from build123d import *

# Parameters (mm, degrees)
SKETCH_1_R          = 11.2
EXTRUDE_1_DEPTH     = 2
SKETCH_2_OUTSIDE_W  = 30.748
SKETCH_2_OUTSIDE_H  = 30.748
CUT_EXTRUDE_1_DEPTH = 2
SKETCH_3_R          = 6.9
EXTRUDE_2_DEPTH     = 13.5
SKETCH_4_R          = 1.2
CUT_EXTRUDE_2_DEPTH = 13.5
FILLET_1_R          = 0.3


with BuildPart() as part:
    # 草图1 → 凸台-拉伸1 (new body)
    with BuildSketch(Plane(origin=(0, 0, 0), x_dir=(1, 0, 0), z_dir=(0, 1, 0))):
        with Locations(Location((0, 0, 0), (0, 0, 270))):
            Circle(SKETCH_1_R)
    extrude(amount=EXTRUDE_1_DEPTH)

    # 草图2 outside → 切除-拉伸1 (cut)
    with BuildSketch(Plane(origin=(0, 2, 0), x_dir=(1, 0, 0), z_dir=(0, 1, 0))):
        Rectangle(SKETCH_2_OUTSIDE_W, SKETCH_2_OUTSIDE_H)
        with BuildLine():
            Line((-8, -7.838367177), (8, -7.838367177))
            ThreePointArc((8, -7.838367177), (11.2, 0), (8, 7.838367177))
            Line((8, 7.838367177), (-8, 7.838367177))
            ThreePointArc((-8, 7.838367177), (-11.2, 0), (-8, -7.838367177))
        make_face(mode=Mode.SUBTRACT)
    extrude(amount=-CUT_EXTRUDE_1_DEPTH, mode=Mode.SUBTRACT)

    # 草图3 → 凸台-拉伸2 (add)
    with BuildSketch(Plane(origin=(0, 2, 0), x_dir=(1, 0, 0), z_dir=(0, 1, 0))):
        with Locations(Location((0, 0, 0), (0, 0, 270))):
            Circle(SKETCH_3_R)
    extrude(amount=EXTRUDE_2_DEPTH)

    # 草图4 → 切除-拉伸2 (cut)
    with BuildSketch(Plane(origin=(0, 2, 0), x_dir=(1, 0, 0), z_dir=(0, 1, 0))):
        with Locations(Location((-8, 5, 0), (0, 0, 270))):
            Circle(SKETCH_4_R)
        with Locations(Location((-8, -5, 0), (0, 0, 270))):
            Circle(SKETCH_4_R)
        with Locations(Location((8, -5, 0), (0, 0, 270))):
            Circle(SKETCH_4_R)
        with Locations(Location((8, 5, 0), (0, 0, 270))):
            Circle(SKETCH_4_R)
    extrude(amount=-CUT_EXTRUDE_2_DEPTH, mode=Mode.SUBTRACT)

    # 圆角1
    fillet_1_edges = [part.edges().sort_by_distance(p)[0] for p in [
        (0, 15.5, -6.9),
    ]]
    fillet(fillet_1_edges, radius=FILLET_1_R)

    # 草图5 → 切除-旋转1 (revolve, cut)
    with BuildSketch(Plane(origin=(0, 15.5, 0), x_dir=(1, 0, 0), z_dir=(0, 1, 0))):
        with BuildLine():
            Line((0, 4.5), (0, -4.5))
            ThreePointArc((0, -4.5), (4.5, 0), (0, 4.5))
        make_face()
    revolve(axis=Axis((0, 15.5, 4.5), (0, 0, -1)), mode=Mode.SUBTRACT)


solid = part.part
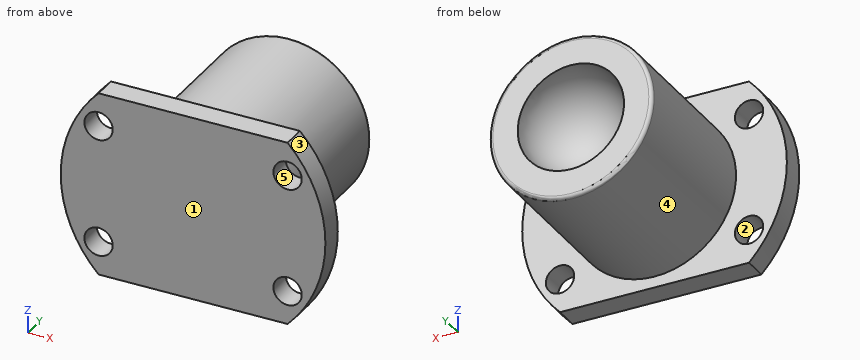
Here's how the part is built. I have some questions about the finished solid (model axes, mm). Face numbers are marked on the shaded views. A direction names the side the tool comes from. Coordinates: 2 decimals unless noted, no trailing zeros. Loops run counter-clockwise (first coordinate to the right, second up) from the corner with the lowest first, then second, coordinate; pieces in that order, holes last.
1. Imagine slicing it at A-A, the plane x = -8.5. Please give me the cut outline in (y, z).
2. Imagine slicing it at B-B, the plane z = 0. Please give me the cut outline in (x, y), and give its area (3 significant figures).
3. If we mould it in two halves opening along X, with no side actions, what happens to the marked faces 1, 2 and 3? For each: pulls with the +X half, pulls with the -X half, needs draft (parallel to the pull), parting line crosses it, or undercut.
4. For the marked faces 4 and 5, which set-ups out of +Z, -Z, +X, -X, +Y, -Y let a thin tool reach every point of the face, with its end or its side?
5. Imagine slicing it at D-D, the plane y = 14. Please give me the cut outline in (x, z).
6. I need wall thicknesses on L1, parallel to X at y = 1.35, z = -5; L2, parallel to Y at x = -1.75, z = 6.75; L3, parallel to X at y = 6.25, z = 0.25. Which ranges of each line are inside material? Lowest first, please.
7. Imagine slicing it at C-C, the plane y = 3. Please give me the cut outline in (x, z).
8. For P1, Ø4, axis at x = 8, z = 5, coming from the +Y side; P2, Ø1.5, axis at x = -2.5, y = 11.5, coming from the +Z side; P3, Ø5, axis at y = 10.5, z = -2.5, coming from the +X side; P4, Ø1.9, axis at x = 8, z = -5, coming from the -Y side, each with a flat end and sliding along its axis, tell me the tip position at first contact or that it passes through.
Taken from the geometry:
1. outline: (0, -7.29) - (2, -7.29) - (2, -6.09) - (0, -6.09) - close; (0, -3.91) - (2, -3.91) - (2, 3.91) - (0, 3.91) - close; (0, 6.09) - (2, 6.09) - (2, 7.29) - (0, 7.29) - close
2. outline: (-11.2, 0) - (11.2, 0) - (11.2, 2) - (6.9, 2) - (6.9, 15.2) arc R0.3 ccw to (6.6, 15.5) - (4.5, 15.5) arc R4.5 cw to (-4.5, 15.5) - (-6.6, 15.5) arc R0.3 ccw to (-6.9, 15.2) - (-6.9, 2) - (-11.2, 2) - close
2. area: 199 mm2
3. face 1: needs draft
3. face 2: undercut
3. face 3: pulls with the +X half
4. face 4: +Y
4. face 5: +Y, -Y
5. outline: circle Ø13.8 at (0, 0); hole circle Ø8.49 at (0, 0)
6. L1: x = -10.02 to -9.2, -6.8 to 6.8, 9.2 to 10.02
6. L2: y = 0 to 2
6. L3: x = -6.9 to 6.9
7. outline: circle Ø13.8 at (0, 0)
8. P1: stops at y = 2
8. P2: stops at z = 6.67
8. P3: stops at x = 6.9
8. P4: passes through
